```python
from build123d import *

# Parameters (mm, degrees)
SKETCH1_R                      = 6.1
THICKNESS_DEPTH                = 3.5
BOTNUTCUT_START                = -2
SKETCH2_R                      = 2.85
BOTNUTCUT_DEPTH                = 2.6
SKETCH3_R                      = 1.55
BOTSCREWCUT_DEPTH              = 2
CUT_EXTRUDE1_START             = -7
CUT_EXTRUDE1_DEPTH             = 7
RAILNUTCUT_START               = -2
RAILNUTCUT_DEPTH               = 2.6
SKETCH7_R                      = 1.55
RAILSCREWCUT_DEPTH             = 2.6
RAILSCREWCUT_DIRECTION_2_REACH = 53.909
RAILNUTHEADCUT_REACH           = 56.409
RAILNUTHEADCUT_START           = -2.5
SKETCH8_R                      = 2.85
SKETCH9_W                      = 7
SKETCH9_H                      = 0.5
MOVEMENTCUT_DEPTH              = 7
SKETCH10_R                     = 4.5
BOSS_EXTRUDE1_DEPTH            = 3.5


with BuildPart() as part:
    # Sketch1 → Thickness (new, symmetric)
    with BuildSketch(Plane.XY):
        with BuildLine():
            Line((-13, -50), (13, -50))
            Line((13, -50), (8.424323952, -3.441041405))
            ThreePointArc((8.424323952, -3.441041405), (0, 9.1), (-8.424323952, -3.441041405))
            Line((-8.424323952, -3.441041405), (-13, -50))
        make_face()
        Circle(SKETCH1_R, mode=Mode.SUBTRACT)
    extrude(amount=THICKNESS_DEPTH, both=True)

    # Sketch2 → BotNutCut (cut)
    with BuildSketch(Plane.XZ.offset(50).offset(BOTNUTCUT_START)):
        with Locations((-7.5, 0)):
            Circle(SKETCH2_R)
        with BuildLine():
            Line((-10.790896534, 2.85), (-10.790896534, 0))
            Line((-10.790896534, 0), (-9.968172361, -1.42500007))
            ThreePointArc((-9.968172361, -1.42500007), (-9.96817242, 1.424999968), (-7.499999995, 2.85))
            Line((-7.499999995, 2.85), (-10.790896534, 2.85))
        make_face()
        with BuildLine():
            Line((-4.209103466, 2.85), (-7.499999995, 2.85))
            ThreePointArc((-7.499999995, 2.85), (-5.484745672, 2.015254324), (-4.65, 0))
            ThreePointArc((-4.65, 0), (-4.747111384, -0.737634237), (-5.031827556, -1.424999925))
            Line((-5.031827556, -1.424999925), (-4.209103466, 0))
            Line((-4.209103466, 0), (-4.209103466, 2.85))
        make_face()
        with BuildLine():
            ThreePointArc((-5.031827556, -1.424999925), (-6.074999963, -2.468172379), (-7.5, -2.85))
            Line((-7.5, -2.85), (-5.854551733, -2.85))
            Line((-5.854551733, -2.85), (-5.031827556, -1.424999925))
        make_face()
        with BuildLine():
            ThreePointArc((-7.5, -2.85), (-8.924999965, -2.468172421), (-9.968172361, -1.42500007))
            Line((-9.968172361, -1.42500007), (-9.145448267, -2.85))
            Line((-9.145448267, -2.85), (-7.5, -2.85))
        make_face()
        with BuildLine():
            ThreePointArc((7.5, -2.85), (6.074999995, -2.468172398), (5.031827593, -1.42499999))
            Line((5.031827593, -1.42499999), (5.854551733, -2.85))
            Line((5.854551733, -2.85), (7.5, -2.85))
        make_face()
        with BuildLine():
            ThreePointArc((9.968172375, -1.425000045), (8.924999978, -2.468172414), (7.5, -2.85))
            Line((7.5, -2.85), (9.145448267, -2.85))
            Line((9.145448267, -2.85), (9.968172375, -1.425000045))
        make_face()
        with BuildLine():
            Line((10.790896534, 2.85), (7.5, 2.85))
            ThreePointArc((7.5, 2.85), (9.515254326, 2.015254326), (10.35, 0))
            ThreePointArc((10.35, 0), (10.252888598, -0.737634304), (9.968172375, -1.425000045))
            Line((9.968172375, -1.425000045), (10.790896534, 0))
            Line((10.790896534, 0), (10.790896534, 2.85))
        make_face()
        with BuildLine():
            Line((4.209103466, 2.85), (4.209103466, 0))
            Line((4.209103466, 0), (5.031827593, -1.42499999))
            ThreePointArc((5.031827593, -1.42499999), (5.031827602, 1.425000005), (7.5, 2.85))
            Line((7.5, 2.85), (4.209103466, 2.85))
        make_face()
        with Locations((7.5, 0)):
            Circle(SKETCH2_R)
    extrude(amount=-BOTNUTCUT_DEPTH, mode=Mode.SUBTRACT)

    # Sketch3 → BotScrewCut (cut)
    with BuildSketch(Plane.XZ.offset(50)):
        with Locations(Location((-7.5, 0, 0), (0, 0, 270))):
            Circle(SKETCH3_R)
        with Locations(Location((7.5, 0, 0), (0, 0, 270))):
            Circle(SKETCH3_R)
    extrude(amount=-BOTSCREWCUT_DEPTH, mode=Mode.SUBTRACT)

    # Sketch5 → Cut-Extrude1 (cut)
    with BuildSketch(Plane.XY.offset(3.5).offset(CUT_EXTRUDE1_START)):
        with BuildLine():
            ThreePointArc((0.5, -6.079473661), (0, -6.1), (-0.5, -6.079473661))
            Line((-0.5, -6.079473661), (-0.5, -12.924568984))
            ThreePointArc((-0.5, -12.924568984), (0, -23.1), (0.5, -12.924568984))
            Line((0.5, -12.924568984), (0.5, -6.079473661))
        make_face()
    extrude(amount=CUT_EXTRUDE1_DEPTH, mode=Mode.SUBTRACT)

    # Sketch6 → RailNutCut (cut)
    with BuildSketch(Plane(origin=(-0.5, 0, 0), x_dir=(0, 0, -1), z_dir=(1, 0, 0)).offset(RAILNUTCUT_START)):
        Polygon((0, -13.290896534), (2.85, -11.645448267), (2.85, -8.354551733), (0, -6.709103466), (-2.85, -6.709103466), (-2.85, -13.290896534), align=None)
    extrude(amount=-RAILNUTCUT_DEPTH, mode=Mode.SUBTRACT)

    # Sketch7 → RailScrewCut (cut)
    with BuildSketch(Plane(origin=(-0.5, 0, 0), x_dir=(0, 0, -1), z_dir=(1, 0, 0))):
        with Locations(Location((0, -10, 0), (0, 0, 270))):
            Circle(SKETCH7_R)
    extrude(amount=-RAILSCREWCUT_DEPTH, mode=Mode.SUBTRACT)

    # RailScrewCut direction 2: up to this plane
    railscrewcut_direction_2_end = Plane(origin=(13, -50, 3.5), z_dir=(-0.9952055153223801, -0.09780583966162733, 0))
    # Sketch7 → RailScrewCut direction 2 (cut, up to the surface)
    with BuildSketch(Plane(origin=(-0.5, 0, 0), x_dir=(0, 0, -1), z_dir=(1, 0, 0)), mode=Mode.PRIVATE) as railscrewcut_direction_2_sk1:
        with Locations(Location((0, -10, 0), (0, 0, 270))):
            Circle(SKETCH7_R)
    railscrewcut_direction_2_tool1 = split(extrude(railscrewcut_direction_2_sk1.sketch, amount=RAILSCREWCUT_DIRECTION_2_REACH, mode=Mode.PRIVATE), bisect_by=railscrewcut_direction_2_end, keep=Keep.BOTH, mode=Mode.PRIVATE)
    add(railscrewcut_direction_2_tool1.solids().sort_by_distance((-0.5, -10, 0))[0], mode=Mode.SUBTRACT)

    # RailNutHeadCut: up to this plane
    railnutheadcut_end = Plane(origin=(13, -50, 3.5), z_dir=(-0.9952055153223801, -0.09780583966162733, 0))
    # Sketch8 → RailNutHeadCut (cut, up to the surface)
    with BuildSketch(Plane.ZY.offset(-0.5).offset(RAILNUTHEADCUT_START), mode=Mode.PRIVATE) as railnutheadcut_sk1:
        with Locations(Location((0, -10, 0), (0, 0, 270))):
            Circle(SKETCH8_R)
    railnutheadcut_tool1 = split(extrude(railnutheadcut_sk1.sketch, amount=-RAILNUTHEADCUT_REACH, mode=Mode.PRIVATE), bisect_by=railnutheadcut_end, keep=Keep.BOTH, mode=Mode.PRIVATE)
    add(railnutheadcut_tool1.solids().sort_by_distance((3, -10, 0))[0], mode=Mode.SUBTRACT)

    # Sketch9 → MovementCut (cut)
    with BuildSketch(Plane.XY.offset(3.5)):
        with Locations((7.5, -18.75)):
            Rectangle(SKETCH9_W, SKETCH9_H)
    extrude(amount=-MOVEMENTCUT_DEPTH, mode=Mode.SUBTRACT)

    # Sketch10 → Boss-Extrude1 (add, symmetric)
    with BuildSketch(Plane.XY):
        with BuildLine():
            Line((-0.5, -13.527864045), (-0.5, -12.924568984))
            ThreePointArc((-0.5, -12.924568984), (-3.780537731, -21.42308844), (5.0009999, -19))
            Line((5.0009999, -19), (4.387482194, -19))
            ThreePointArc((4.387482194, -19), (-3.356217727, -20.997632828), (-0.5, -13.527864045))
        make_face()
        with Locations((0, -18)):
            Circle(SKETCH10_R)
    extrude(amount=BOSS_EXTRUDE1_DEPTH, both=True)


solid = part.part
```
Source: CAD feature listing. Evaluate the final solid. Frame: model axes, mm. A direction names the side the tool comes from. Round coordinates to 2 decimals unless told otherwise and drop trailing zeros. Loops run counter-clockwise (first coordinate to the right, second up) from the corner with the lowest first, then second, coordinate; pieces in that order, holes last. Notation, with made-up numbers: M 86,8.5 L 143,8.5 A22 cw 143,20.5 Z; hole C 58.5,68.5 d3. An arc over 180 degrees is marked long. Put each result on its own line as item: value.
(1) Section A-A, the plane y = 0. Return loops of the section in (x, z).
Solutions:
outline: M -9.1,-3.5 L -6.1,-3.5 L -6.1,3.5 L -9.1,3.5 Z; M 6.1,-3.5 L 9.1,-3.5 L 9.1,3.5 L 6.1,3.5 Z
(2) Access query for faces 1 (the face through (-8, -45.4, 0)), 2 (the face through (7, -19, 0)), 3 (the face through (6.13, -12.633, -1.092)), 4 (the face through (0.5, -8, 0)). Directions: +Z, -Z, +X, -X, +Y, -Y. A direction counts if a zero-diameter tool reaches every point of the face in a straight line with its end or side. Return the directions, or none.
Solutions:
face 1: none
face 2: +Z, -Z, +X
face 3: +X
face 4: +Z, -Z
(3) Section C-C, the plane y = -10. Return loops of the section in (x, z), and give its area (3 significant figures).
Solutions:
outline: M -9.07,-3.5 L -0.5,-3.5 L -0.5,-1.55 L -2.5,-1.55 L -2.5,-2.85 L -5.1,-2.85 L -5.1,2.85 L -2.5,2.85 L -2.5,1.55 L -0.5,1.55 L -0.5,3.5 L -9.07,3.5 Z; M 0.5,-3.5 L 9.07,-3.5 L 9.07,-2.85 L 3,-2.85 L 3,-1.55 L 0.5,-1.55 Z; M 0.5,1.55 L 3,1.55 L 3,2.85 L 9.07,2.85 L 9.07,3.5 L 0.5,3.5 Z
area: 56.6 mm²
(4) Section D-D, the plane y = -34. Return loops of the section in (x, z), and give its area (3 significant figures).
Solutions:
outline: M -11.43,-3.5 L 11.43,-3.5 L 11.43,3.5 L -11.43,3.5 Z
area: 160 mm²
(5) Section B-B, the plane x = 7.5. Return loops of the section in (y, z).
Solutions:
outline: M -50,-3.5 L -19,-3.5 L -19,3.5 L -50,3.5 L -50,1.55 L -48,1.55 L -48,2.85 L -45.4,2.85 L -45.4,-2.85 L -48,-2.85 L -48,-1.55 L -50,-1.55 Z; M -18.5,-3.5 L 5.15,-3.5 L 5.15,3.5 L -18.5,3.5 Z; hole C -10,0 d5.7
(6) Pull-direction query (X, two-part tool) for faces 5 (the face through (-4, -10, 2.85)), 6 (the face through (-4.209, -47, 1)), 7 (the face through (-1.49, -8.77, 0.94)), 8 (the face through (9.34, -12.75, 1.6)); classes: released by +X, released by -X, zero draft, split by the parting line, or undercut.
Solutions:
face 5: undercut
face 6: undercut
face 7: zero draft
face 8: released by +X
(7) First-contact query: pin 1 (2 mm diameter, centred on y = -8.5, z = 1, fed in from +X); pin 2 (4 mm diameter, centred on y = -40, z = 2, fed in from -X); pin 3 (2 mm diameter, centred on y = -47, z = 1, fed in from -X). Flat tips, straight axial feed; report the tip coordinate or a pass-through.
Solutions:
pin 1: x = 3
pin 2: x = -12.21
pin 3: x = -12.8
(8) Ray query, line 1 (Z direction, x = -3, y = -8.5); line 2 (Y direction, x = 6.5, z = 0.5); line 3 (X direction, y = 0, z = -0.5). Return the intervals inside material, ascending. Write a range as [from, to].
Solutions:
line 1: [-3.5, -2.85], [2.85, 3.5]
line 2: [-45.4, -19], [-18.5, -12.81], [-7.19, 6.37]
line 3: [-9.1, -6.1], [6.1, 9.1]
